CAD build for the part. Positions are in the model's coordinates, mm. Face numbers are marked on the shaded views. A direction names the side the tool comes from. Round coordinates to 2 decimals unless told otherwise and drop trailing zeros. Order: outer loops, then holes, each group sorted by start corner. A loop starts at its lowest first (then second) coordinate and runs counter-clockwise, first axis right, second up. Notation, with made-up numbers: (46, 60.25) -> (101, 60.25) arc R21 ccw to (101, 93.25) -> close; hole circle Ø6 at (10, 69). An arc over 180 degrees is marked (long way). Return JSON: item names as keys, results as strings. Group by question number.
Q1. Cut at A-A (z = 6). Write the cut outline in (x, y).
Q2. Which spindle directions (+Z, -Z, +X, -X, +Y, -Y) get a long thin tool onto all of the face, cutting with end or side? Do the marked faces 1 and 2. Say none if no direction does.
Q3. Cut at C-C (y = 19). Write the cut outline in (x, z), then the cut area to 3 significant figures.
Q4. Flat gauge pins, fed straight in: pin 1 (6 mm diameter, centred on x = 29, y = 1.5, fed in from +Z); pin 2 (2 mm diameter, centred on x = -31.5, y = -42.5, fed in from +Z); pin 3 (3 mm diameter, centred on x = -9.5, y = 39, fed in from +Z). Where does each tip first touch, or does it go through?
Q5. Mould opens along Y. For the marked faces 3, 4 and 5 say: +Y half, -Y half, draft (parallel to the pull), parting line (faces both ways), or undercut.
Q6. Cut at B-B (x = 5). Write the cut outline in (y, z).
Q7. Probe line 1 along X through (y, z) = (-14.5, 5); line 2 along Y through (x, z) = (10, 8); line 3 along Z through (x, y) = (-27.5, 14). List the from-to ranges inside material, lowest first.
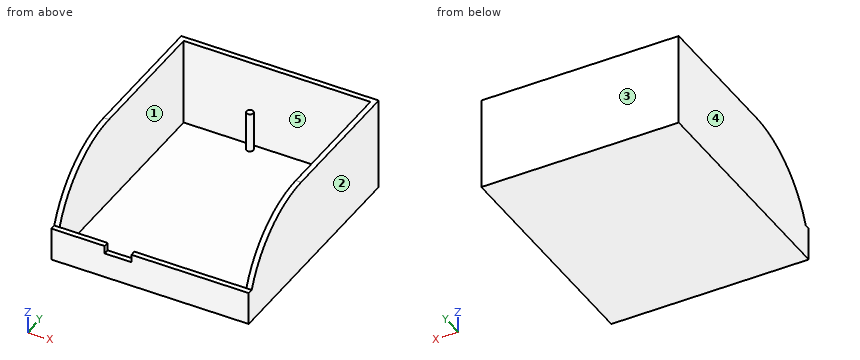
from build123d import *

# Parameters (mm, degrees)
F0_W      = 74
F0_H      = 87.5
F1_DEPTH  = 34
F2_W      = 70
F2_H      = 83.5
F4_DEPTH  = 33
F3_W      = 2
F3_H      = 22.5
F5_DEPTH  = 74
F8_DEPTH  = 15
F9_DEPTH  = 1
F6_W      = 10
F6_H      = 3
F10_DEPTH = 4


with BuildPart() as f1:
    # F0 (on Top) → F1 (new body)
    with BuildSketch(Plane.XY):
        Rectangle(F0_W, F0_H)
    extrude(amount=F1_DEPTH)

    # F2 (on face) → F4 (cut)
    with BuildSketch(Plane.XY.offset(34)):
        Rectangle(F2_W, F2_H)
    extrude(amount=-F4_DEPTH, mode=Mode.SUBTRACT)

    # F3 (on face) → F5 (cut)
    with BuildSketch(Plane(origin=(-37, 0, 0), x_dir=(0, -1, 0), z_dir=(-1, 0, 0))):
        with BuildLine():
            Line((41.75, 34), (8.5, 34))
            ThreePointArc((8.5, 34), (28.573692, 27.846401), (41.75, 11.5))
            Line((41.75, 11.5), (41.75, 34))
        make_face()
        with Locations((42.75, 22.75)):
            Rectangle(F3_W, F3_H)
    extrude(amount=-F5_DEPTH, mode=Mode.SUBTRACT)

    # F7 (on face) → F8 (join)
    with BuildSketch(Plane.XY.offset(1)):
        with BuildLine():
            ThreePointArc((-7.5, 39.25), (-7.866117, 40.133883), (-8.75, 40.5))
            Line((-8.75, 40.5), (-8.75, 39.25))
            Line((-8.75, 39.25), (-10, 39.25))
            ThreePointArc((-10, 39.25), (-8.75, 38), (-7.5, 39.25))
        make_face()
        with BuildLine():
            Line((-8.75, 39.25), (-8.75, 40.5))
            ThreePointArc((-8.75, 40.5), (-9.633883, 40.133883), (-10, 39.25))
            Line((-10, 39.25), (-8.75, 39.25))
        make_face()
    extrude(amount=F8_DEPTH)

    # F0 (on Top) → F9 (join)
    with BuildSketch(Plane.XY):
        Rectangle(F0_W, F0_H)
    extrude(amount=-F9_DEPTH)

    # F6 (on face) → F10 (cut)
    with BuildSketch(Plane.XZ.offset(43.75)):
        with Locations((-12, 10)):
            Rectangle(F6_W, F6_H)
    extrude(amount=-F10_DEPTH, mode=Mode.SUBTRACT)


solid = f1.part
Solution:
{
 "1": {"outline": "(-37, -43.75) -> (37, -43.75) -> (37, 43.75) -> (-37, 43.75) -> close; (-10, 39.25) arc R1.25 ccw to (-7.5, 39.25) arc R1.25 ccw to (-8.75, 40.5) arc R1.25 ccw to start; hole (-35, -41.75) -> (35, -41.75) -> (35, 41.75) -> (-35, 41.75) -> close"},
 "2": {"face 1": "+Z", "face 2": "+Z, -Z, +X, +Y, -Y"},
 "3": {"outline": "(-37, -1) -> (37, -1) -> (37, 34) -> (35, 34) -> (35, 1) -> (-35, 1) -> (-35, 34) -> (-37, 34) -> close", "area": "280 mm²"},
 "4": {"pin 1": "stops at z = 1", "pin 2": "stops at z = 11.5", "pin 3": "stops at z = 16"},
 "5": {"face 3": "+Y half", "face 4": "draft", "face 5": "undercut"},
 "6": {"outline": "(-43.75, -1) -> (43.75, -1) -> (43.75, 34) -> (41.75, 34) -> (41.75, 1) -> (-41.75, 1) -> (-41.75, 11.5) -> (-43.75, 11.5) -> close"},
 "7": {"line 1": "x = -37 to -35, 35 to 37", "line 2": "y = -43.75 to -41.75, 41.75 to 43.75", "line 3": "z = -1 to 1"}
}
